The model under review builds one solid part; all positions refer to its coordinate system, in mm. A direction names the side the tool comes from. Coordinates: 2 decimals unless noted, no trailing zeros. Loops run counter-clockwise (first coordinate to the right, second up) from the corner with the lowest first, then second, coordinate; pieces in that order, holes last. Notation, with made-up numbers: (-33, 71.5) - (25, 71.5) arc R13 ccw to (25, 87.5) - close; hole circle Ø6 at (38.25, -39.75). An arc over 180 degrees is marked (long way). Answer in a Markdown table with one row per item. Add a question column.
(1) For P1, Ø1.5, axis at x = 4.5, y = 13, coming from the +Z side, flat-tipped, find the tip position at first contact; note if it passes through.
(2) We need section B-B on y = 17.5. Write out the cut boundary in (x, z), plus the area to 3 significant figures.
(3) We need section A-A on x = 4. Write out the cut boundary in (y, z), plus the area to 3 significant figures.
(4) Machinability: for faces 4 (the flat face through (0, 9, 4)), 5 (the flat face through (18, 3, -1)), 6 (the flat face through (18, 41, 8)), 7 (the flat face through (-2, 18.5, 4)), 8 (the flat face through (18, 37, -2.5)), which of the approach directions +Z, -Z, +X, -X, +Y, -Y give a long, thin tool a straight path to every point of the face, cutting with its end or side? Answer none if there is none.
(5) Mouldability with a two-part tool opening along X and no side actions: class faces 1 (the flat face through (38, 21, 4)), 2 (the flat face through (18, 36.5, -1)), 3 (the flat face through (-5, 19, -1)) as +X half, -X half, draft (parallel to the pull), parting line (faces both ways), or undercut.
(6) We need section D-D on x = 35. Write out the cut boundary in (y, z), plus the area to 3 significant figures.
(7) We need section C-C on z = 5.5. Write out the cut boundary in (x, y), plus the area to 3 significant figures.
(8) For line 1 along Y through (x, z) = (31, 3.75); line 2 along Y through (x, z) = (39.5, 4.5); line 3 along X through (y, z) = (31, -0.25), list the stretches that pass through material, from the lowest coordinate up.
from build123d import *

# Parameters (mm, degrees)
BOSS_EXTRUDE1_DEPTH   = 8
BOSS_EXTRUDE1_2_DEPTH = 8
SKETCH2_W             = 46
SKETCH2_H             = 49.5
SKETCH2_W_2           = 30
SKETCH2_H_2           = 33.5
BOSS_EXTRUDE2_DEPTH   = 2.5


with BuildPart() as part:
    # Sketch1 → Boss-Extrude1 (new body)
    with BuildSketch(Plane.XY):
        Polygon((-5, 21), (0, 21), (0, 39.5), (36, 39.5), (36, 21), (41, 21), (41, 44.5), (-5, 44.5), align=None)
    extrude(amount=BOSS_EXTRUDE1_DEPTH)



with BuildPart() as body_2:
    # Sketch1 → Boss-Extrude1 2 (new body)
    with BuildSketch(Plane.XY):
        Polygon((36, 0), (0, 0), (0, 18.5), (-5, 18.5), (-5, -5), (41, -5), (41, 18.5), (36, 18.5), align=None)
    extrude(amount=BOSS_EXTRUDE1_2_DEPTH)


with BuildPart() as part_1:
    add(part.part)

    add(body_2.part)  # Boss-Extrude2 merges body 2
    # Sketch2 → Boss-Extrude2 (add)
    with BuildSketch(Plane(origin=(0, 0, 0), x_dir=(-1, 0, 0), z_dir=(0, 0, -1))):
        with Locations((-18, 19.75)):
            Rectangle(SKETCH2_W, SKETCH2_H)
        with Locations((-18, 19.75)):
            Rectangle(SKETCH2_W_2, SKETCH2_H_2, mode=Mode.SUBTRACT)
    extrude(amount=BOSS_EXTRUDE2_DEPTH)


solid = part_1.part
Outcome:
| question | item | result |
|---|---|---|
| 1 | P1 | through |
| 2 | outline | (-5, -2.5) - (3, -2.5) - (3, 0) - (0, 0) - (0, 8) - (-5, 8) - close; (33, -2.5) - (41, -2.5) - (41, 8) - (36, 8) - (36, 0) - (33, 0) - close |
| 2 | area | 120 mm² |
| 3 | outline | (-5, -2.5) - (3, -2.5) - (3, 0) - (0, 0) - (0, 8) - (-5, 8) - close; (36.5, -2.5) - (44.5, -2.5) - (44.5, 8) - (39.5, 8) - (39.5, 0) - (36.5, 0) - close |
| 3 | area | 120 mm² |
| 4 | face 4 | +Z |
| 4 | face 5 | +Z, -Z |
| 4 | face 6 | +Z, +X, -X, +Y, -Y |
| 4 | face 7 | +Z, +X, -X |
| 4 | face 8 | -Z, +X, -X, +Y, -Y |
| 5 | face 1 | draft |
| 5 | face 2 | undercut |
| 5 | face 3 | -X half |
| 6 | outline | (-5, -2.5) - (44.5, -2.5) - (44.5, 8) - (39.5, 8) - (39.5, 0) - (0, 0) - (0, 8) - (-5, 8) - close |
| 6 | area | 204 mm² |
| 7 | outline | (-5, -5) - (41, -5) - (41, 18.5) - (36, 18.5) - (36, 0) - (0, 0) - (0, 18.5) - (-5, 18.5) - close; (-5, 21) - (0, 21) - (0, 39.5) - (36, 39.5) - (36, 21) - (41, 21) - (41, 44.5) - (-5, 44.5) - close |
| 7 | area | 830 mm² |
| 8 | line 1 | -5 to 0, 39.5 to 44.5 |
| 8 | line 2 | -5 to 18.5, 21 to 44.5 |
| 8 | line 3 | -5 to 3, 33 to 41 |
